from build123d import *

# Parameters (mm, degrees)
CUBE001_W      = 30
CUBE001_H      = 30
CUBE001_DEPTH  = 1
CYLINDER_R     = 10
CYLINDER_DEPTH = 2
CUBE_W         = 40
CUBE_H         = 40
CUBE_DEPTH     = 6


with BuildPart() as cube001:
    # cube001 → cube001 (new body)
    with BuildSketch(Plane(origin=(-15, -15, 2), x_dir=(1, 0, 0), z_dir=(0, 0, 1))):
        with Locations((15, 15)):
            Rectangle(CUBE001_W, CUBE001_H)
    extrude(amount=CUBE001_DEPTH)


with BuildPart() as union:
    # cylinder → cylinder (new body)
    with BuildSketch(Plane.XY.offset(1)):
        Circle(CYLINDER_R)
    extrude(amount=CYLINDER_DEPTH)

    # union: union cube001
    add(cube001.part)


with BuildPart() as difference:
    # cube → cube (new body)
    with BuildSketch(Plane(origin=(-20, -20, -3), x_dir=(1, 0, 0), z_dir=(0, 0, 1))):
        with Locations((20, 20)):
            Rectangle(CUBE_W, CUBE_H)
    extrude(amount=CUBE_DEPTH)

    # difference: cut union
    add(union.part, mode=Mode.SUBTRACT)


solid = difference.part
Input: part model. Units: mm. Frame: model coordinates. A direction names the side the tool comes from. Coordinates: 2 decimals unless noted, no trailing zeros. Order: outer loops, then holes, each group sorted by start corner. A loop starts at its lowest first (then second) coordinate and runs counter-clockwise, first axis right, second up.
1. Draft query along X for faces 1 (the flat face through (20, 0, 0)), 2 (the flat face through (-15, -0.2, 2.5)), 3 (the flat face through (-18, 0, 3)). Return one class per face: +X half, -X half, draft (parallel to the pull), parting line (faces both ways), or undercut.
Checked values:
face 1: +X half
face 2: undercut
face 3: draft
2. Cut plane C-C, the plane x = -14.5. Return loops of the section in (y, z), plus the area to 3 significant figures.
Checked values:
outline: (-20, -3) - (20, -3) - (20, 3) - (15, 3) - (15, 2) - (-15, 2) - (-15, 3) - (-20, 3) - close
area: 210 mm2
3. Ray query, line 1 along Y through (x, z) = (6, 2.2); line 2 along X through (y, z) = (0, 1.35). Return the intervals inside material, ascending.
Checked values:
line 1: y = -20 to -15, 15 to 20
line 2: x = -20 to -10, 10 to 20
4. Contact query for flat-ended pins moving along their axis: P1, Ø6, axis at x = -1.5, y = 4, coming from the +Z side; P2, Ø15, axis at x = 3.5, y = -7, coming from the +Z side. Output: stop coordinate, or through.
Checked values:
P1: stops at z = 1
P2: stops at z = 2
5. Cut plane A-A, the plane x = 0. Return loops of the section in (y, z), plus the area to 3 significant figures.
Checked values:
outline: (-20, -3) - (20, -3) - (20, 3) - (15, 3) - (15, 2) - (10, 2) - (10, 1) - (-10, 1) - (-10, 2) - (-15, 2) - (-15, 3) - (-20, 3) - close
area: 190 mm2
6. Access query for faces 4 (the flat face through (-0.2, 10.2, 2)), 5 (the flat face through (-20, 0, 0)). Directions: +Z, -Z, +X, -X, +Y, -Y. A direction counts if a zero-diameter tool reaches every point of the face in a straight line with its end or side. Return the directions, or none.
Checked values:
face 4: +Z
face 5: +Z, -Z, -X, +Y, -Y
